Print and shaded views of the part. All mm, measured from the part's lowest x, y and z. Give positions to 0.01 mm unless a question says otherwise; leave off trailing zeros. Loops run counter-clockwise (first coordinate to the right, second up) from the corner with the lowest first, then second, coordinate; pieces in that order, holes last.
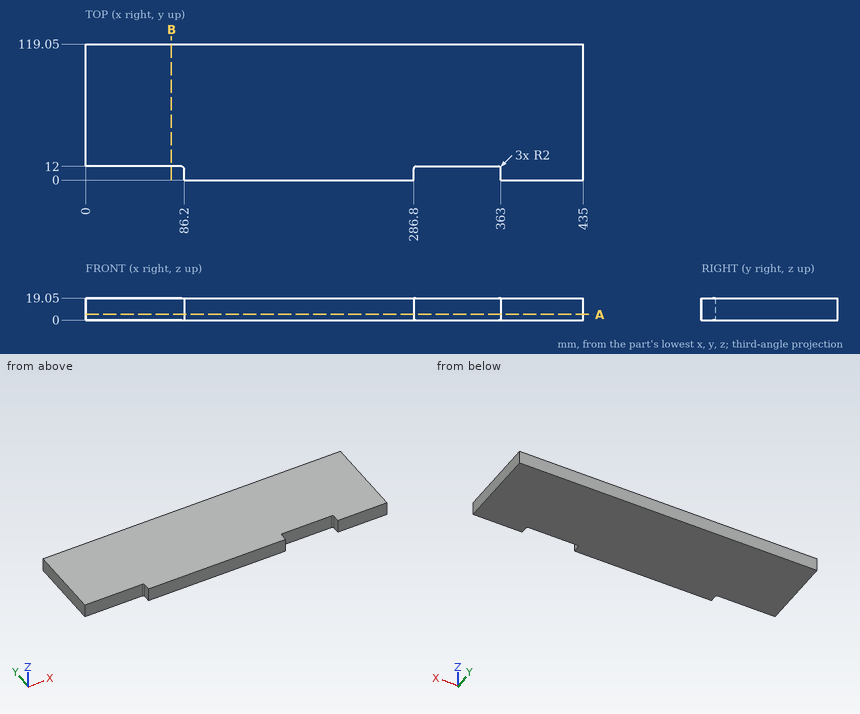
1. Saw through at A-A, the plane z = 5. List the corners of the cut face in (x, y).
Responses:
outline: (0, 12) - (84.2, 12) arc R2 cw to (86.2, 10) - (86.2, 0) - (286.8, 0) - (286.8, 10) arc R2 cw to (288.8, 12) - (361, 12) arc R2 cw to (363, 10) - (363, 0) - (435, 0) - (435, 119.05) - (0, 119.05) - close
2. Saw through at B-B, the plane x = 75. List the corners of the cut face in (y, z), and give its area (3 significant figures).
Responses:
outline: (12, 0) - (119.05, 0) - (119.05, 19.05) - (12, 19.05) - close
area: 2,040 mm2
3. Probe line 1 along Y through (x, z) = (72.5, 13). List the from-to ranges inside material, lowest first.
Responses:
line 1: y = 12 to 119.05
4. Drop flat-ended pins along their axis: pin 1 (9.5 mm diameter, centred on x = 342.5, z = 11, fed in from -Y); pin 2 (6 mm diameter, centred on y = 21.5, z = 3, fed in from -X); pin 3 (11 mm diameter, centred on y = 2.5, z = 14, fed in from -X). Give the stop position or say it passes through.
Responses:
pin 1: stops at y = 12
pin 2: stops at x = 0
pin 3: stops at x = 86.2
